```python
from build123d import *

# Parameters (mm, degrees)
F0_W      = 30
F0_H      = 30
F0_W_2    = 5
F0_H_2    = 5
F1_DEPTH  = 5
F2_DEPTH  = 35
F3_DEPTH  = 65
F4_R      = 2.1
F6_DEPTH  = 25
F5_R      = 2.1
F7_DEPTH  = 25
F8_R      = 3.75
F8_R_2    = 2.1
F9_DEPTH  = 4
F10_DEPTH = 25
F11_START = 4
F11_DEPTH = 4
F13_SIZE  = 10


# Not quite as in the source:
# - a fillet or chamfer that OpenCascade refuses, or shapes differently, is made with other operations: its cross-section is extruded or revolved along the edge and cut away or added


with BuildPart() as f1:
    # F0 (on Top) → F1 (new body)
    with BuildSketch(Plane.XY):
        with BuildLine():
            Line((-35, 30), (-30, 30))
            Line((-30, 30), (-30, 35))
            ThreePointArc((-30, 35), (-33.5355339059, 33.5355339059), (-35, 30))
        make_face()
        with Locations((15, 15)):
            Rectangle(F0_W, F0_H)
        with BuildLine():
            Line((0, 35), (0, 30))
            Line((0, 30), (30, 30))
            ThreePointArc((30, 30), (28.5355339059, 33.5355339059), (25, 35))
            Line((25, 35), (0, 35))
        make_face()
        with Locations((-15, -15)):
            Rectangle(F0_W, F0_H)
        with Locations((-32.5, 15)):
            Rectangle(F0_W_2, F0_H)
        with BuildLine():
            Line((30, 0), (0, 0))
            Line((0, 0), (0, -30))
            ThreePointArc((0, -30), (21.2132034356, -21.2132034356), (30, 0))
        make_face()
        with Locations((-15, 32.5)):
            Rectangle(F0_W, F0_H_2)
        with BuildLine():
            Line((-30, -30), (-30, 0))
            Line((-30, 0), (-35, 0))
            Line((-35, 0), (-35, -25))
            ThreePointArc((-35, -25), (-33.5355339059, -28.5355339059), (-30, -30))
        make_face()
        with Locations((-15, 15)):
            Rectangle(F0_W, F0_H)
    extrude(amount=F1_DEPTH)

    # F0 (on Top) → F2 (join)
    with BuildSketch(Plane.XY):
        with BuildLine():
            Line((-30, -30), (-30, 0))
            Line((-30, 0), (-35, 0))
            Line((-35, 0), (-35, -25))
            ThreePointArc((-35, -25), (-33.5355339059, -28.5355339059), (-30, -30))
        make_face()
        with Locations((-32.5, 15)):
            Rectangle(F0_W_2, F0_H)
        with BuildLine():
            Line((-35, 30), (-30, 30))
            Line((-30, 30), (-30, 35))
            ThreePointArc((-30, 35), (-33.5355339059, 33.5355339059), (-35, 30))
        make_face()
        with BuildLine():
            Line((0, 35), (0, 30))
            Line((0, 30), (30, 30))
            ThreePointArc((30, 30), (28.5355339059, 33.5355339059), (25, 35))
            Line((25, 35), (0, 35))
        make_face()
        with Locations((-15, 32.5)):
            Rectangle(F0_W, F0_H_2)
    extrude(amount=F2_DEPTH)

    # F0 (on Top) → F3 (join)
    with BuildSketch(Plane.XY):
        with Locations((-15, 32.5)):
            Rectangle(F0_W, F0_H_2)
        with BuildLine():
            Line((-35, 30), (-30, 30))
            Line((-30, 30), (-30, 35))
            ThreePointArc((-30, 35), (-33.5355339059, 33.5355339059), (-35, 30))
        make_face()
        with Locations((-32.5, 15)):
            Rectangle(F0_W_2, F0_H)
    extrude(amount=F3_DEPTH)

    # F4 (on face) → F6 (cut)
    with BuildSketch(Plane(origin=(0, 35, 0), x_dir=(-1, 0, 0), z_dir=(0, 1, 0))):
        with Locations((15, 17.5)):
            Circle(F4_R)
        with Locations((6.3242963515, 17.5)):
            Circle(F4_R)
        with Locations((-6.6132452339, 17.5)):
            Circle(F4_R)
        with Locations((-20.042758435, 17.5)):
            Circle(F4_R)
        with Locations((15, 42.3774681985)):
            Circle(F4_R)
        with Locations((15, 57.9239465296)):
            Circle(F4_R)
    extrude(amount=-F6_DEPTH, mode=Mode.SUBTRACT)

    # F5 (on face) → F7 (cut)
    with BuildSketch(Plane(origin=(-35, 0, 0), x_dir=(0, -1, 0), z_dir=(-1, 0, 0))):
        with Locations((21.9386201352, 17.5704155117)):
            Circle(F5_R)
        with Locations((7.1015073918, 17.5704155117)):
            Circle(F5_R)
        with Locations((-15, 17.5704155117)):
            Circle(F5_R)
        with Locations((-6.9537893869, 17.5704155117)):
            Circle(F5_R)
        with Locations((-15, 41.8734140694)):
            Circle(F5_R)
        with Locations((-15, 56.0644082725)):
            Circle(F5_R)
    extrude(amount=-F7_DEPTH, mode=Mode.SUBTRACT)

    # F8 (on face) → F9 (cut)
    with BuildSketch(Plane.XY):
        with Locations((-15.0563415678, 14.7660031606)):
            Circle(F8_R)
        with Locations((-15.0563415678, 14.7660031606)):
            Circle(F8_R_2, mode=Mode.SUBTRACT)
        with Locations((0, 14.7660031606)):
            Circle(F8_R)
        with Locations((0, 14.7660031606)):
            Circle(F8_R_2, mode=Mode.SUBTRACT)
        with Locations((15.0742138934, 14.7859862541)):
            Circle(F8_R)
        with Locations((15.0742138934, 14.7859862541)):
            Circle(F8_R_2, mode=Mode.SUBTRACT)
        with Locations((14.9396037335, -15.2109106032)):
            Circle(F8_R)
        with Locations((14.9396037335, -15.2109106032)):
            Circle(F8_R_2, mode=Mode.SUBTRACT)
        with Locations((0, -15.1403872296)):
            Circle(F8_R)
        with Locations((0, -15.1403872296)):
            Circle(F8_R_2, mode=Mode.SUBTRACT)
        with Locations((-14.9904824793, -15.1403872296)):
            Circle(F8_R)
        with Locations((-14.9904824793, -15.1403872296)):
            Circle(F8_R_2, mode=Mode.SUBTRACT)
        with Locations((-15.0563415678, 0)):
            Circle(F8_R)
        with Locations((-15.0563415678, 0)):
            Circle(F8_R_2, mode=Mode.SUBTRACT)
    extrude(amount=F9_DEPTH, mode=Mode.SUBTRACT)

    # F8 (on face) → F10 (cut)
    with BuildSketch(Plane.XY):
        with Locations((-14.9904824793, -15.1403872296)):
            Circle(F8_R_2)
        with BuildLine():
            Line((0, -17.2403872296), (0, -13.0403872296))
            ThreePointArc((0, -13.0403872296), (-2.1, -15.1403872296), (0, -17.2403872296))
        make_face()
        with BuildLine():
            ThreePointArc((2.1, -15.1403872296), (1.4849242405, -13.6554629891), (0, -13.0403872296))
            Line((0, -13.0403872296), (0, -17.2403872296))
            ThreePointArc((0, -17.2403872296), (1.4849242405, -16.6253114701), (2.1, -15.1403872296))
        make_face()
        with Locations((14.9396037335, -15.2109106032)):
            Circle(F8_R_2)
        with Locations((15.0742138934, 14.7859862541)):
            Circle(F8_R_2)
        with Locations((0, 14.7660031606)):
            Circle(F8_R_2)
        with Locations((-15.0563415678, 14.7660031606)):
            Circle(F8_R_2)
        with BuildLine():
            Line((-17.1563415678, 0), (-12.9563415678, 0))
            ThreePointArc((-12.9563415678, 0), (-15.0563415678, 2.1), (-17.1563415678, 0))
        make_face()
        with BuildLine():
            ThreePointArc((-17.1563415678, 0), (-15.0563415678, -2.1), (-12.9563415678, 0))
            Line((-12.9563415678, 0), (-17.1563415678, 0))
        make_face()
    extrude(amount=F10_DEPTH, mode=Mode.SUBTRACT)

    # F8 (on face) → F11 (join)
    with BuildSketch(Plane.XY.offset(F11_START)):
        with Locations((-14.9904824793, -15.1403872296)):
            Circle(F8_R)
        with Locations((-14.9904824793, -15.1403872296)):
            Circle(F8_R_2, mode=Mode.SUBTRACT)
        with Locations((14.9396037335, -15.2109106032)):
            Circle(F8_R)
        with Locations((14.9396037335, -15.2109106032)):
            Circle(F8_R_2, mode=Mode.SUBTRACT)
        with Locations((-15.0563415678, 14.7660031606)):
            Circle(F8_R)
        with Locations((-15.0563415678, 14.7660031606)):
            Circle(F8_R_2, mode=Mode.SUBTRACT)
        with Locations((15.0742138934, 14.7859862541)):
            Circle(F8_R)
        with Locations((15.0742138934, 14.7859862541)):
            Circle(F8_R_2, mode=Mode.SUBTRACT)
    extrude(amount=F11_DEPTH)

    # F12: chamfer of 2 on 4 edges, made by hand

    # F12_s1 → F12_t2 (revolve, cut)
    with BuildSketch(Plane.XZ.offset(-14.7660031606)):
        Polygon((-11.3063415678, 6), (-13.3063415678, 8), (-11.3063415678, 8), align=None)
    revolve(axis=Axis((-15.0563415678, 14.7660031606, 8), (0, 0, 1)), mode=Mode.SUBTRACT)

    # F12_s3 → F12_t4 (revolve, cut)
    with BuildSketch(Plane.XZ.offset(-14.7859862541)):
        Polygon((18.8242138934, 6), (16.8242138934, 8), (18.8242138934, 8), align=None)
    revolve(axis=Axis((15.0742138934, 14.7859862541, 8), (0, 0, 1)), mode=Mode.SUBTRACT)

    # F12_s5 → F12_t6 (revolve, cut)
    with BuildSketch(Plane.XZ.offset(15.2109106032)):
        Polygon((18.6896037335, 6), (16.6896037335, 8), (18.6896037335, 8), align=None)
    revolve(axis=Axis((14.9396037335, -15.2109106032, 8), (0, 0, 1)), mode=Mode.SUBTRACT)

    # F12_s7 → F12_t8 (revolve, cut)
    with BuildSketch(Plane.XZ.offset(15.1403872296)):
        Polygon((-11.2404824793, 6), (-13.2404824793, 8), (-11.2404824793, 8), align=None)
    revolve(axis=Axis((-14.9904824793, -15.1403872296, 8), (0, 0, 1)), mode=Mode.SUBTRACT)

    # F13
    f13_edges = [f1.edges().sort_by_distance(p)[0] for p in [
        (-32.5, 0, 65),
        (0, 32.5, 65),
        (-32.5, 0, 35),
        (0, 32.5, 35),
    ]]
    chamfer(f13_edges, length=F13_SIZE)


solid = f1.part
```
Design review of the part built by this model. Coordinates are the model's own, in mm. A direction names the side the tool comes from. Coordinates: 2 decimals unless noted, no trailing zeros. Loops run counter-clockwise (first coordinate to the right, second up) from the corner with the lowest first, then second, coordinate; pieces in that order, holes last.
Q1. To check wall thickness, follow line 1 (Y direction, x = -0.5, z = 23); line 2 (X direction, y = 0, z = 4.65); line 3 (Z direction, x = -18.5, y = 2.5). State the ranges of each line that lie inside material, in increasing order.
Reported:
line 1: y = 30 to 35
line 2: x = -35 to -17.16, -12.96 to 30
line 3: z = 0 to 5
Q2. We need section A-A on x = 6. State the section outline as (y, z) points, and give its area (3 significant figures).
Reported:
outline: (-29.39, 0) - (35, 0) - (35, 15.49) - (30, 15.49) - (30, 5) - (-29.39, 5) - close; (30, 19.51) - (35, 19.51) - (35, 39) - (30, 39) - close
area: 472 mm2
Q3. Tool access review of faces 4 (the face through (-33, 0, 50)), 5 (the face through (13.273, -16.489, 5.799)), 6 (the face through (11.96, -17.49, 5.49)), 7 (the face through (-15, -30, 2)), 8 (the face through (2, 13, 4)): name each direction out of +Z, -Z, +X, -X, +Y, -Y from which nothing blocks a thin tool from reaching the whole face with its end or side.
Reported:
face 4: +Z, +X, -X, -Y
face 5: +Z, -Z
face 6: +Z
face 7: +Z, -Z, +X, -X, -Y
face 8: -Z
Q4. We need section C-C on y = 21. State the section outline as (x, z) points, and give its area (3 significant figures).
Reported:
outline: (-35, 0) - (30, 0) - (30, 5) - (-30, 5) - (-30, 65) - (-35, 65) - close
area: 625 mm2
Q5. We need section B-B on z = 38.5. State the section outline as (x, y) points.
Reported:
outline: (-35, -6.5) - (-30, -6.5) - (-30, 30) - (6.5, 30) - (6.5, 35) - (-30, 35) arc R5 ccw to (-35, 30) - close
Q6. For pin 1 (3.5 mm diameter, centred on y = -7.1, z = 17.57, fed in from -X); pin 2 (5.5 mm diameter, centred on x = 6.61, z = 17.5, fed in from -Y); pin 3 (3 mm diameter, centred on y = 3, z = 38, fed in from +X); pin 4 (5 mm diameter, centred on x = 14.94, y = -15.21, fed in from +Z), all flat-tipped, find the tip position at first contact; note any pin that passes through.
Reported:
pin 1: passes through
pin 2: stops at y = 30
pin 3: stops at x = -30
pin 4: stops at z = 7.65
Q7. The part is to be moulded in two halves that separate along X. For faces 1 (the face through (-18.737, -14.976, 1.972)), 2 (the face through (17, 13, 4)), 3 (the face through (-32.5, 6, 15.7)), say which applies: +X half, -X half, draft (parallel to the pull), parting line (faces both ways), or undercut.
Reported:
face 1: undercut
face 2: undercut
face 3: draft
Q8. We need section D-D on y = 7. State the section outline as (x, z) points.
Reported:
outline: (-35, 0) - (30, 0) - (30, 5) - (-30, 5) - (-30, 15.47) - (-35, 15.47) - close; (-35, 19.67) - (-30, 19.67) - (-30, 62) - (-35, 62) - close
